CAD build for the part. Positions are in the model's coordinates, mm. A direction names the side the tool comes from. Round coordinates to 2 decimals unless told otherwise and drop trailing zeros. Write each loop counter-clockwise with the first axis right and the second up, starting at its lowest first coordinate (ties: lowest second). Pieces come first, ordered by that corner, then holes. Notation, with made-up numbers: (26.5, 65.5) -> (49.5, 65.5) arc R17 ccw to (49.5, 94.5) -> close; hole circle Ø8 at (-22, 44). An arc over 180 degrees is marked (long way). Put each result on its own line as item: value. Start each with the question number.
1. Drill centre lines: line 1 (Y direction, x = -134.5, z = 1); line 2 (Y direction, x = -149, z = 0); line 3 (X direction, y = 2, z = 33). Where is each one in solid material? Low to high. Write a range as from..to.
2. 3-axis set-ups, long thin cutter, end or side, ignore diameter. For faces 4 (the flat face through (-152, -37.408, 0)), 5 (the flat face through (191.319, -3, -32)), 6 (the flat face through (196.249, -20.646, -29.307)), 7 (the flat face through (-152, 30.592, 0)), 8 (the cylindrical face through (196.25, -19.23, 20.64)): which of +Z, -Z, +X, -X, +Y, -Y reach the whole face in a straight line?
3. Flat gauge pins, fed straight in: P1, Ø12, axis at y = 49.5, z = -1, coming from the +X side; P2, Ø12, axis at x = 173, z = 19, coming from the +Y side; P3, Ø8, axis at x = -24.5, y = 50, coming from the -Z side. Where does each tip first touch, or does it go through?
4. Saw through at B-B on z = 0. State how many separate pieces and enclosed holes the cut face has, and give its area (3 significant figures).
5. Pull direction Z, two halves, no side cores. Call faces 1 (the flat face through (-8, 86.592, 0)), 2 (the conical face through (225.9, 22.84, -5.83)), 3 (the conical face through (-23.543, 86.404, -15.44)): pulls with the +Z half, pulls with the -Z half, needs draft (parallel to the pull), parting line crosses it, or undercut.
6. Saw through at C-C on x = 96. List the corners of the cut face in (y, z), and give its area (3 significant figures).
7. Saw through at A-A on x = 146.5. List the corners of the cut face in (y, z), and give its area (3 significant figures).
from build123d import *

# Parameters (mm, degrees)
SKETCH2_R           = 13.003199109
BOSS_EXTRUDE1_DEPTH = 5
BOSS_EXTRUDE2_START = -5
SKETCH3_R           = 13.003199109
BOSS_EXTRUDE2_DEPTH = 5
CHAMFER1_SIZE       = 1.5
CUT_EXTRUDE1_REACH  = 139.423
SKETCH4_R           = 4
CHAMFER2_SIZE       = 1.5
SKETCH7_R           = 5
CUT_EXTRUDE2_DEPTH  = 10
CUT_EXTRUDE2_DRAFT  = 14
SKETCH7_2_R         = 5
CUT_EXTRUDE3_DEPTH  = 10
CUT_EXTRUDE3_DRAFT  = -7
SCALE1_SCALE        = 2


with BuildPart() as part:
    # Sketch1 → Revolve-Thin1 (revolve)
    with BuildSketch(Plane.XY, mode=Mode.PRIVATE) as revolve_thin1_sk:
        Polygon((-94, 15.001980763), (-69, 15.875), (-24.426145366, 15.875), (-3, 7), (0, 7), (67.41231775, 15.875), (110, 15.875), (135, 15.001980763), (134.930201007, 13.003199109), (109.96508987, 13.875), (67.543404676, 13.875), (0.131086926, 5), (-3.397824735, 5), (-24.823970101, 13.875), (-68.96508987, 13.875), (-93.930201007, 13.003199109), align=None)
    revolve(revolve_thin1_sk.sketch.rotate(Axis((-94, 0, 0), (1, 0, 0)), 90), axis=Axis((-94, 0, 0), (1, 0, 0)))

    # Sketch2 → Boss-Extrude1 (add)
    with BuildSketch(Plane(origin=(-69, 0, 0), x_dir=(0, 0, -1), z_dir=(1, 0, 0))):
        Polygon((19.629909152, 0), (9.814954576, 17), (-9.814954576, 17), (-19.629909152, 0), (-9.814954576, -17), (9.814954576, -17), align=None)
        Circle(SKETCH2_R, mode=Mode.SUBTRACT)
    extrude(amount=BOSS_EXTRUDE1_DEPTH)

    # Sketch3 → Boss-Extrude2 (add)
    with BuildSketch(Plane(origin=(110, 0, 0), x_dir=(0, 0, -1), z_dir=(1, 0, 0)).offset(BOSS_EXTRUDE2_START)):
        Polygon((19.629909152, 0), (9.814954576, 17), (-9.814954576, 17), (-19.629909152, 0), (-9.814954576, -17), (9.814954576, -17), align=None)
        Circle(SKETCH3_R, mode=Mode.SUBTRACT)
    extrude(amount=BOSS_EXTRUDE2_DEPTH)

    # Chamfer1
    chamfer1_edges = [part.edges().sort_by_distance(p)[0] for p in [
        (135, 0, -15.001980763),
        (-94, 0, -15.001980763),
    ]]
    chamfer(chamfer1_edges, length=CHAMFER1_SIZE)

    # Sketch4 → Cut-Extrude1 (cut, up to next)
    with BuildSketch(Plane(origin=(0, 0, 0), x_dir=(1, 0, 0), z_dir=(0, 1, 0)), mode=Mode.PRIVATE) as cut_extrude1_sk1:
        with Locations(Location((0, 0, 0), (0, 0, 90))):
            Circle(SKETCH4_R)
    cut_extrude1_tool1 = extrude(cut_extrude1_sk1.sketch, amount=CUT_EXTRUDE1_REACH, mode=Mode.PRIVATE) & part.part
    add(cut_extrude1_tool1.solids().sort_by_distance((0, 0, 0))[0], mode=Mode.SUBTRACT)

    # Sketch5 → Revolve3 (revolve)
    with BuildSketch(Plane.XY, mode=Mode.PRIVATE) as revolve3_sk:
        Polygon((-4, 0), (-8, 1.656854249), (-8, 33), (-9.5, 33), (-9.5, 45), (-5, 45), (-5, 10.414213562), (-4, 10), align=None)
    revolve(revolve3_sk.sketch.rotate(Axis((0, 0, 0), (0, 1, 0)), 270), axis=Axis((0, 0, 0), (0, 1, 0)))

    # Chamfer2
    chamfer2_edges = [part.edges().sort_by_distance(p)[0] for p in [
        (0, 33, 9.5),
        (0, 45, 9.5),
    ]]
    chamfer(chamfer2_edges, length=CHAMFER2_SIZE - 0.0001)  # a hair under: the kernel refuses the full size


with BuildPart() as cut_extrude2_tool:
    # Sketch7 → Cut-Extrude2 (with draft: the straight prism first)
    with BuildSketch(Plane(origin=(0, 0, 0), x_dir=(0, 0, -1), z_dir=(1, 0, 0))):
        Circle(SKETCH7_R)
    extrude(amount=-CUT_EXTRUDE2_DEPTH)
    # Cut-Extrude2: the draft: its side faces are tilted about the plane it starts from
    cut_extrude2_sides = [cut_extrude2_tool.faces().sort_by_distance(p)[0] for p in [
        (-5, 0, 5),
    ]]
    draft(cut_extrude2_sides, Plane(origin=(0, 0, 0), x_dir=(0, 0, -1), z_dir=(1, 0, 0)), CUT_EXTRUDE2_DRAFT)


with BuildPart() as part_1:
    add(part.part)

    # Cut-Extrude2: cut by cut_extrude2_tool
    add(cut_extrude2_tool.part, mode=Mode.SUBTRACT)


with BuildPart() as cut_extrude3_tool:
    # Sketch7<2> → Cut-Extrude3 (with draft: the straight prism first)
    with BuildSketch(Plane(origin=(0, 0, 0), x_dir=(0, 0, -1), z_dir=(1, 0, 0))):
        Circle(SKETCH7_2_R)
    extrude(amount=CUT_EXTRUDE3_DEPTH)
    # Cut-Extrude3: the draft: its side faces are tilted about the plane it starts from
    cut_extrude3_sides = [cut_extrude3_tool.faces().sort_by_distance(p)[0] for p in [
        (5, 0, 5),
    ]]
    draft(cut_extrude3_sides, Plane(origin=(0, 0, 0), x_dir=(0, 0, -1), z_dir=(1, 0, 0)), CUT_EXTRUDE3_DRAFT)


with BuildPart() as part_2:
    add(part_1.part)

    # Cut-Extrude3: cut by cut_extrude3_tool
    add(cut_extrude3_tool.part, mode=Mode.SUBTRACT)


with BuildPart() as part_3:
    # Scale1: scaled about (18.680604314, 3.407991009, 5.57e-07)
    add(part_2.part.scale(SCALE1_SCALE).moved(Location((-18.680604314, -3.407991009, -5.57e-07))))


solid = part_3.part
Return value:
1. line 1: y = -35.14..-31.14, 24.32..28.33
1. line 2: y = -37.41..-29.41, 22.6..30.59
1. line 3: x = -156.68..-146.68, 191.32..201.32
2. face 4: +Z, -Z, +X, -X, -Y
2. face 5: none
2. face 6: -Z, +X, -X, -Y
2. face 7: +Z, -Z, -X, +Y
2. face 8: +X
3. P1: stops at x = -2.68
3. P2: stops at y = 25.56
3. P3: stops at z = -15.9
4. separate pieces: 3
4. enclosed holes: 0
4. area: 4,790 mm^2
5. face 1: needs draft
5. face 2: undercut
5. face 3: parting line crosses it
6. outline: circle Ø58.2 at (-3.41, 0); hole circle Ø50.13 at (-3.41, 0)
6. area: 686 mm^2
7. outline: circle Ø63.5 at (-3.41, 0); hole circle Ø55.5 at (-3.41, 0)
7. area: 748 mm^2
